Design review of the part built by this model. Coordinates are the model's own, in mm. Face numbers are marked on the shaded views. A direction names the side the tool comes from. Give positions to 0.01 mm unless a question says otherwise; leave off trailing zeros. Loops run counter-clockwise (first coordinate to the right, second up) from the corner with the lowest first, then second, coordinate; pieces in that order, holes last. Notation, with made-up numbers: M -1.75,-31 L 53.25,-31 A15 ccw 53.25,-12 Z; hole C -2,26.5 d2. An arc over 180 degrees is marked long. Use CSV: the item, a comma, the result in double quotes.
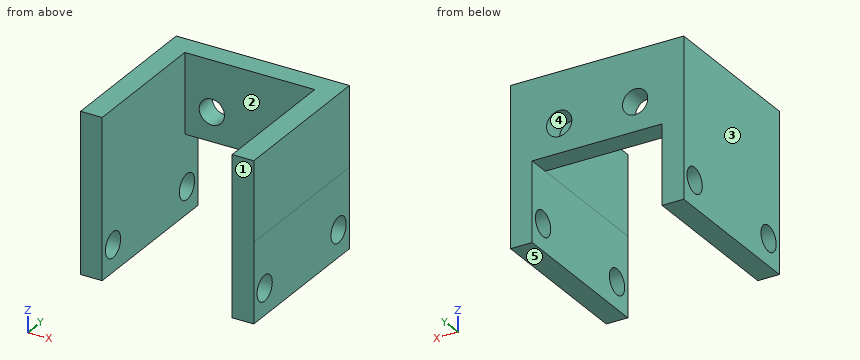
from build123d import *

# Parameters (mm, degrees)
SKETCH_1_W                  = 22
SKETCH_1_H                  = 21.992162459
EXTRUDE_1_DEPTH             = 2.999999998
EXTRUDE_2_DEPTH             = 10.99608123
SKETCH_3_W                  = 3
SKETCH_3_H                  = 22
EXTRUDE_3_DEPTH             = 10.996081229
HOLE_WIZARD_3_5_3_5_1_D     = 3.5
HOLE_WIZARD_3_5_3_5_1_DEPTH = 22.000025
HOLE_WIZARD_3_5_3_5_2_D     = 3.5
HOLE_WIZARD_3_5_3_5_2_DEPTH = 3
HOLE_WIZARD_3_5_3_5_3_D     = 3.5


with BuildPart() as part:
    # 스케치1 → 보스-돌출1 (new body)
    with BuildSketch(Plane(origin=(-11.99726579, 0, 0), x_dir=(0, -1, 0), z_dir=(-1, 0, 0))):
        with Locations((11, -15.30483348)):
            Rectangle(SKETCH_1_W, SKETCH_1_H)
    extrude(amount=-EXTRUDE_1_DEPTH)

    # 스케치2 → 보스-돌출2 (add)
    with BuildSketch(Plane.XY.offset(-4.30875225)):
        Polygon((12, 0), (-8.99726579, 0), (-8.99726579, -2.999999996), (9, -2.999999996), (9, -21.999999998), (12, -21.999999998), align=None)
    extrude(amount=-EXTRUDE_2_DEPTH)

    # 스케치3 → 보스-돌출3 (add)
    with BuildSketch(Plane(origin=(0, 0, -15.30483348), x_dir=(-1.0, 0, 5.95310697820905e-12), z_dir=(-5.95310697820905e-12, 0, -1.0))):
        with Locations((-10.5, -11)):
            Rectangle(SKETCH_3_W, SKETCH_3_H)
    extrude(amount=EXTRUDE_3_DEPTH)

    # Ø3.5 (3.5) 지름 구멍1
    with Locations(Plane(origin=(0, 0, 0), x_dir=(1, 0, 0), z_dir=(0, 1, 0))):
        with Locations((-5.258745872, 11.300890987), (5.258745872, 11.300890987)):
            Hole(HOLE_WIZARD_3_5_3_5_1_D / 2, depth=HOLE_WIZARD_3_5_3_5_1_DEPTH)

    # Ø3.5 (3.5) 지름 구멍2
    with Locations(Plane.ZY.offset(-9)):
        with Locations((-22.606276953, -19.5), (-22.606276953, -2.5)):
            Hole(HOLE_WIZARD_3_5_3_5_2_D / 2, depth=HOLE_WIZARD_3_5_3_5_2_DEPTH)

    # Ø3.5 (3.5) 지름 구멍3 (through all)
    with Locations(Plane(origin=(-8.997265792, 0, 0), x_dir=(0, 0, -1), z_dir=(1, 0, 0))):
        with Locations((22.606276953, -19.5), (22.606276953, -2.5)):
            Hole(HOLE_WIZARD_3_5_3_5_3_D / 2)


solid = part.part
(1) We need section D-D on y = -19.5. State the section outline as (x, z) points, then the cut area to 3 significant figures.
A:
outline,"M -12,-26.3 L -9,-26.3 L -9,-24.36 L -12,-24.36 Z; M -12,-20.86 L -9,-20.86 L -9,-4.31 L -12,-4.31 Z; M 9,-26.3 L 12,-26.3 L 12,-24.36 L 9,-24.36 Z; M 9,-20.86 L 12,-20.86 L 12,-4.31 L 9,-4.31 Z"
area,"111 mm²"
(2) We need section B-B on x = -5. State the section outline as (y, z) points.
A:
outline,"M -3,-15.3 L 0,-15.3 L 0,-13.03 L -3,-13.03 Z; M -3,-9.57 L 0,-9.57 L 0,-4.31 L -3,-4.31 Z"
(3) Machinability: for the marked faces 1 and 2, which of the approach directions +Z, -Z, +X, -X, +Y, -Y give a long, thin tool a straight path to every point of the face, cutting with its end or side? Answer none if there is none.
A:
face 1,"+Z, -Z, +X, -X, -Y"
face 2,"+Z, -Z, -Y"
(4) Wall thickness on line 1 along X through (y, z) = (-5.25, -19); line 2 along Z through (x, y) = (10.75, -19.5); line 3 along Z through (x, y) = (7.5, -1.25): over which ranges is each line inside the solid? List them lowest first. Write a range as [from, to].
A:
line 1,"[-12, -9], [9, 12]"
line 2,"[-26.3, -24.36], [-20.86, -4.31]"
line 3,"[-15.3, -4.31]"
(5) The part is to be moulded in two halves that separate along X. For the marked faces 3, 4 and 5, say which applies: released by +X, released by -X, zero draft, split by the parting line, or undercut.
A:
face 3,"released by -X"
face 4,"undercut"
face 5,"zero draft"
(6) Clearance check with flat-ended pins moving along their axes: P1, Ø5.5, axis at x = -5.26, z = -11.3, coming from the -Y side; P2, Ø1.5, axis at x = 0, y = -2, coming from the -Z side. State where each tip first meets the part, or that it passes through.
A:
P1,"y = -3"
P2,"z = -15.3"
(7) We need section A-A on y = -7.25. State the section outline as (x, z) points, then the cut area to 3 significant figures.
A:
outline,"M -12,-26.3 L -9,-26.3 L -9,-4.31 L -12,-4.31 Z; M 9,-26.3 L 12,-26.3 L 12,-4.31 L 9,-4.31 Z"
area,"132 mm²"
(8) We need section C-C on z = -22. State the section outline as (x, y) points, then the cut area to 3 significant figures.
A:
outline,"M -12,-22 L -9,-22 L -9,-21.14 L -12,-21.14 Z; M -12,-17.86 L -9,-17.86 L -9,-4.14 L -12,-4.14 Z; M -12,-0.86 L -9,-0.86 L -9,0 L -12,0 Z; M 9,-22 L 12,-22 L 12,-21.14 L 9,-21.14 Z; M 9,-17.86 L 12,-17.86 L 12,-4.14 L 9,-4.14 Z; M 9,-0.86 L 12,-0.86 L 12,0 L 9,0 Z"
area,"92.6 mm²"
